Print and shaded views of the part. All mm, measured from the part's lowest x, y and z. Round coordinates to 2 decimals unless told otherwise and drop trailing zeros. Write each loop counter-clockwise with the first axis right and the second up, starting at its lowest first coordinate (ties: lowest second). Pieces come first, ordered by that corner, then holes. Notation, with made-up numbers: (22, 53) -> (56, 53) arc R27 cw to (56, 69) -> close; hole circle Ø5 at (0, 14.5). An arc over 180 degrees is marked (long way). Return JSON: item names as keys, results as strings. Group by question number.
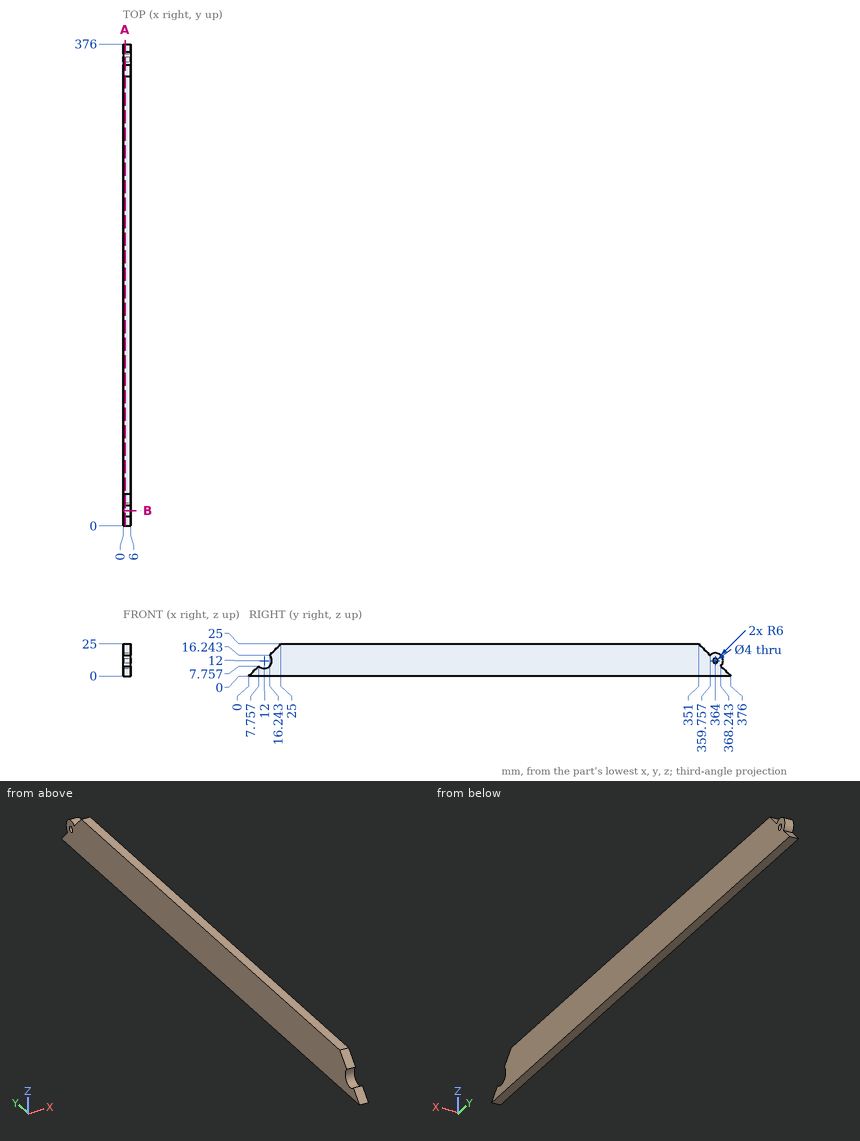
Item 1: Flat gauge pin, fed straight in: P1, Ø2, axis at x = 3, z = 9, coming from the +Y side. Where does the tip first touch, or does it go through?
Item 2: Wall check: L1, parallel to Z at x = 3.7, y = 364; L2, parallel to Y at x = 4, z = 12; L3, parallel to Y at x = 0.8, z = 4. Give the ranges that are in metal, low to high.
Item 3: Cut at A-A (x = 1.55). Write the cut outline in (y, z), then the cut area to 3 significant figures.
Item 4: Cut at B-B (y = 12). Write the cut outline in (x, z), then the cut area to 3 significant figures.
Checks:
{
 "1": {"P1": "stops at y = 369.66"},
 "2": {"L1": "z = 0 to 10, 14 to 18", "L2": "y = 18 to 362, 366 to 370", "L3": "y = 4 to 372"},
 "3": {"outline": "(0, 0) -> (376, 0) -> (368.24, 7.76) arc R6 ccw to (359.76, 16.24) -> (351, 25) -> (25, 25) -> (16.24, 16.24) arc R6 cw to (7.76, 7.76) -> close; hole circle Ø4 at (364, 12)", "area": "8,760 mm2"},
 "4": {"outline": "(0, 0) -> (6, 0) -> (6, 6) -> (0, 6) -> close", "area": "36.0 mm2"}
}
